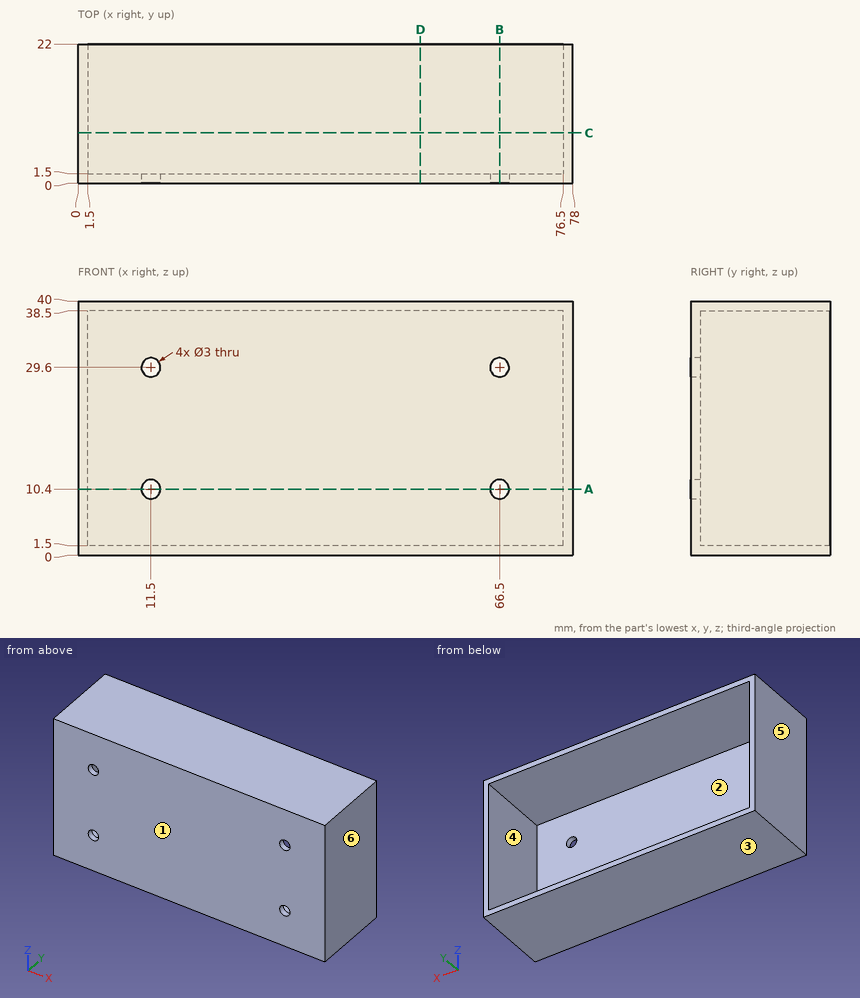
The drawing under review shows one solid part. Ordinate dimensions are in mm from its lowest x, y, z. A direction names the side the tool comes from. Give positions to 0.01 mm unless a question says otherwise; leave off trailing zeros. Write each loop counter-clockwise with the first axis right and the second up, starting at its lowest first coordinate (ties: lowest second). Pieces come first, ordered by that corner, then holes.
1. Draft analysis for pull direction X (two halves, no side actions). For the marked faces 3, 4, 5 and 6, state which applies: +X half, -X half, draft (parallel to the pull), parting line (faces both ways), or undercut.
2. Add section D-D, the plane x = 54. Write out the cut boundary in (y, z).
3. Add section C-C, the plane y = 8. Write out the cut boundary in (x, z), plus the area to 3 significant figures.
4. Tool access review of the marked faces 1 and 2: name each direction out of +Z, -Z, +X, -X, +Y, -Y from which nothing blocks a thin tool from reaching the whole face with its end or side.
5. Add section B-B, the plane x = 66.5. Write out the cut boundary in (y, z), plus the area to 4 significant figures.
6. For P1, Ø4, axis at x = 11.5, z = 10.4, coming from the +Y side, flat-tipped, find the tip position at first contact; note if it passes through.
7. Wall thickness on L1, parallel to X at y = 0.6, z = 29.6; L2, parallel to Z at x = 51.5, y = 14.5; L3, parallel to X at y = 14.75, z = 10.5: over which ranges is each line inside the solid? List them lowest first.
8. Add section A-A, the plane z = 10.4. Write out the cut boundary in (x, y).
Worked answers:
1. face 3: draft
1. face 4: undercut
1. face 5: -X half
1. face 6: +X half
2. outline: (0, 0) - (22, 0) - (22, 1.5) - (1.5, 1.5) - (1.5, 38.5) - (22, 38.5) - (22, 40) - (0, 40) - close
3. outline: (0, 0) - (78, 0) - (78, 40) - (0, 40) - close; hole (1.5, 1.5) - (76.5, 1.5) - (76.5, 38.5) - (1.5, 38.5) - close
3. area: 345 mm2
4. face 1: +Z, -Z, +X, -X, -Y
4. face 2: +Y
5. outline: (0, 0) - (22, 0) - (22, 1.5) - (1.5, 1.5) - (1.5, 8.9) - (0, 8.9) - close; (0, 11.9) - (1.5, 11.9) - (1.5, 28.1) - (0, 28.1) - close; (0, 31.1) - (1.5, 31.1) - (1.5, 38.5) - (22, 38.5) - (22, 40) - (0, 40) - close
5. area: 112.5 mm2
6. P1: stops at y = 1.5
7. L1: x = 0 to 10, 13 to 65, 68 to 78
7. L2: z = 0 to 1.5, 38.5 to 40
7. L3: x = 0 to 1.5, 76.5 to 78
8. outline: (0, 0) - (10, 0) - (10, 1.5) - (1.5, 1.5) - (1.5, 22) - (0, 22) - close; (13, 0) - (65, 0) - (65, 1.5) - (13, 1.5) - close; (68, 0) - (78, 0) - (78, 22) - (76.5, 22) - (76.5, 1.5) - (68, 1.5) - close
